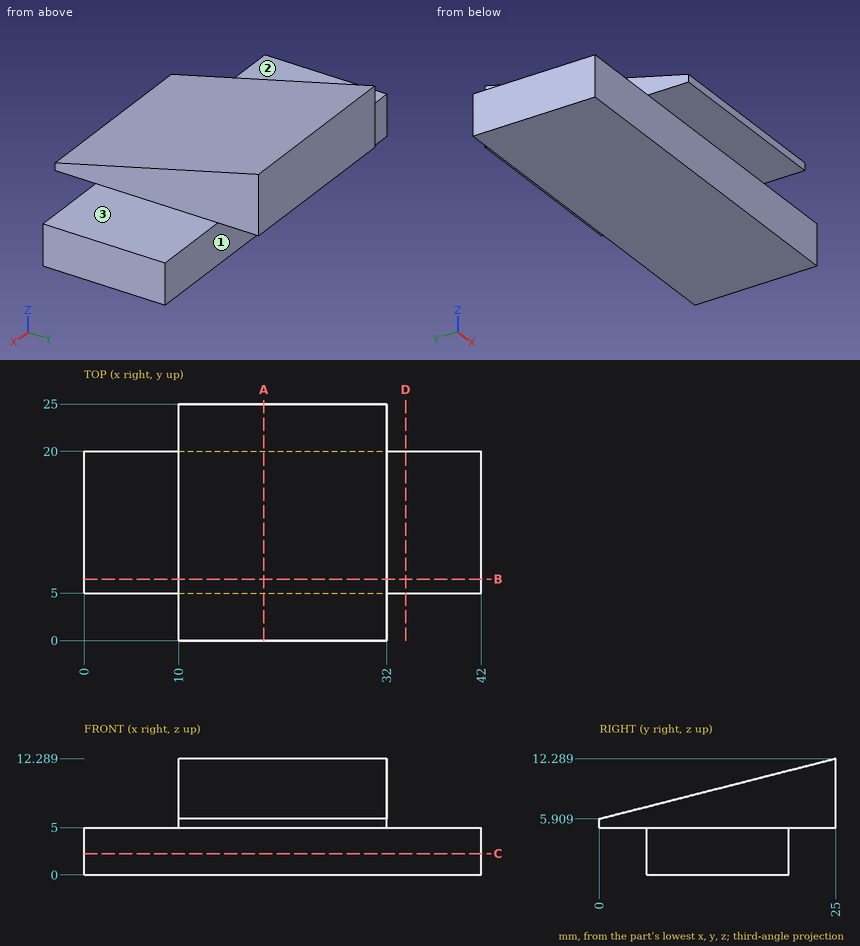
Verification items for this drawing (mm, ordinates from the low corner). A direction names the side the tool comes from. Coordinates: 2 decimals unless noted, no trailing zeros. Loops run counter-clockwise (first coordinate to the right, second up) from the corner with the lowest first, then second, coordinate; pieces in that order, holes last.
Item 1: Sectioned sample at C-C, the plane z = 2.25. Record the boundary of the cut face in (x, y).
Item 2: Sectioned sample at A-A, the plane x = 19. Record the boundary of the cut face in (y, z).
Item 3: Sectioned sample at B-B, the plane y = 6.5. Record the boundary of the cut face in (x, z).
Item 4: Sectioned sample at D-D, the plane x = 34. Record the boundary of the cut face in (y, z), then the cut area to 3 significant figures.
Item 5: Thickness scan on line 1 (Y direction, x = 27.5, z = 3.75); line 2 (Z direction, x = 37, y = 11.5); line 3 (X direction, y = 22, z = 10). Record the ranges inside material, lowest first.
Item 6: Access from +Z, -Z, +X, -X, +Y, -Y to the whole of each face (thin tool, end or side, straight path). Record for the marked faces 1, 2 and 3.
Item 7: Go/stop test with flat-tipped pins: pin 1 Ø5.5 at (x, y) = (16, 2) entering from -Z; pin 2 Ø4 at (x, y) = (10.5, 21.5) entering from +Z; pin 3 Ø3 at (x, y) = (36.5, 13) entering from +Z; pin 4 Ø3 at (x, z) = (36, 8) entering from -Y. Record where each tip stops, or that it passes through.
Check result:
1. outline: (0, 5) - (42, 5) - (42, 20) - (0, 20) - close
2. outline: (0, 5) - (5, 5) - (5, 0) - (20, 0) - (20, 5) - (25, 5) - (25, 12.29) - (0, 5.91) - close
3. outline: (0, 0) - (42, 0) - (42, 5) - (32, 5) - (32, 7.57) - (10, 7.57) - (10, 5) - (0, 5) - close
4. outline: (5, 0) - (20, 0) - (20, 5) - (5, 5) - close
4. area: 75.0 mm2
5. line 1: y = 5 to 20
5. line 2: z = 0 to 5
5. line 3: x = 10 to 32
6. face 1: -Z, +X, -X, +Y
6. face 2: +Z, -X, +Y, -Y
6. face 3: +Z, +X, +Y, -Y
7. pin 1: stops at z = 5
7. pin 2: stops at z = 11.91
7. pin 3: stops at z = 5
7. pin 4: passes through
